Part model, mm, in its own coordinate system. A direction names the side the tool comes from. Round coordinates to 2 decimals unless told otherwise and drop trailing zeros. Write each loop counter-clockwise with the first axis right and the second up, starting at its lowest first coordinate (ties: lowest second). Pieces come first, ordered by that corner, then holes. Notation, with made-up numbers: M 7,20.5 L 17,20.5 A17 cw 17,52.5 Z; hole C 56,35.5 d8. An arc over 180 degrees is marked long. One line per question, with ' | ' between items. Start each with the question number.
1) Tool access for faces 5 (the face through (75, 3, -51)), 6 (the face through (49, 3, 0)): list every direction of +Z, -Z, +X, -X, +Y, -Y with a clear straight run to the whole face (end or side of a thin tool).
2) Drop flat-ended pins along their axis: pin 1 Ø11 at (x, z) = (87.7, -12.7) entering from -Y; pin 2 Ø6.5 at (x, z) = (87.7, -38.1) entering from -Y. Give the stop position or say it passes through.
3) Saw through at A-A (z = -58.5). List the corners of the cut face in (x, y), plus the area to 3 significant figures.
4) Mould opens along X. For faces 1 (the face through (25.4, 3, -50)), 2 (the face through (49, 0, -22)), 3 (the face through (100.4, 3, -38)), 4 (the face through (90.933, 3.219, -11.359)) say: pulls with the +X half, pulls with the -X half, needs draft (parallel to the pull), parting line crosses it, or undercut.
5) Saw through at C-C (y = 2). Give the number of separate pieces and of enclosed holes in the cut face, plus the area to 3 significant figures.
6) Saw through at B-B (x = 37.5). List the corners of the cut face in (y, z).
7) Saw through at D-D (z = -12.7). List the corners of the cut face in (x, y), plus the area to 3 significant figures.
8) Wall check: probe 1 along Z at (x, y) = (87.7, 2.25); probe 2 along X at (y, z) = (3.75, -38.1); probe 3 along X at (y, z) = (5.25, -12.7). Give the ranges that are in metal, low to high. Write a range as [from, to].
```python
from build123d import *

# Parameters (mm, degrees)
BOSS_EXTRUDE1_DEPTH = 6.35
SKETCH2_R           = 3.5
CUT_EXTRUDE1_DEPTH  = 6.35


with BuildPart() as part:
    # Sketch1 → Boss-Extrude1 (new body)
    with BuildSketch(Plane(origin=(0, 0, 0), x_dir=(1, 0, 0), z_dir=(0, 1, 0))):
        Polygon((0, 76.2), (0, 0), (25.4, 0), (75, 0), (100.4, 0), (100.4, 76.2), (75, 76.2), (75, 25.4), (25.4, 25.4), (25.4, 76.2), align=None)
    extrude(amount=BOSS_EXTRUDE1_DEPTH)

    # Sketch2 → Cut-Extrude1 (cut)
    with BuildSketch(Plane(origin=(0, 6.35, 0), x_dir=(1, 0, 0), z_dir=(0, 1, 0))):
        with Locations((12.7, 12.7)):
            Circle(SKETCH2_R)
        with Locations((12.7, 38.1)):
            Circle(SKETCH2_R)
        with Locations((12.7, 63.5)):
            Circle(SKETCH2_R)
        with Locations((87.7, 63.5)):
            Circle(SKETCH2_R)
        with Locations((87.7, 38.1)):
            Circle(SKETCH2_R)
        with Locations((87.7, 12.7)):
            Circle(SKETCH2_R)
        with Locations((37.5, 12.7)):
            Circle(SKETCH2_R)
        with Locations((62.9, 12.7)):
            Circle(SKETCH2_R)
    extrude(amount=-CUT_EXTRUDE1_DEPTH, mode=Mode.SUBTRACT)


solid = part.part
```
Answer key:
1) face 5: -Z, +Y, -Y | face 6: +Z, +X, -X, +Y, -Y
2) pin 1: stops at y = 0 | pin 2: passes through
3) outline: M 0,0 L 25.4,0 L 25.4,6.35 L 0,6.35 Z; M 75,0 L 100.4,0 L 100.4,6.35 L 75,6.35 Z | area: 323 mm2
4) face 1: undercut | face 2: needs draft | face 3: pulls with the +X half | face 4: undercut
5) separate pieces: 1 | enclosed holes: 8 | area: 4,820 mm2
6) outline: M 0,-25.4 L 6.35,-25.4 L 6.35,-16.2 L 0,-16.2 Z; M 0,-9.2 L 6.35,-9.2 L 6.35,0 L 0,0 Z
7) outline: M 0,0 L 9.2,0 L 9.2,6.35 L 0,6.35 Z; M 16.2,0 L 34,0 L 34,6.35 L 16.2,6.35 Z; M 41,0 L 59.4,0 L 59.4,6.35 L 41,6.35 Z; M 66.4,0 L 84.2,0 L 84.2,6.35 L 66.4,6.35 Z; M 91.2,0 L 100.4,0 L 100.4,6.35 L 91.2,6.35 Z | area: 460 mm2
8) probe 1: z = [-76.2, -67], [-60, -41.6], [-34.6, -16.2], [-9.2, 0] | probe 2: x = [0, 9.2], [16.2, 25.4], [75, 84.2], [91.2, 100.4] | probe 3: x = [0, 9.2], [16.2, 34], [41, 59.4], [66.4, 84.2], [91.2, 100.4]
